The listing builds one solid part. Answer for the finished solid, in the listing's coordinates (mm). Give positions to 0.01 mm unless a question says otherwise; leave off trailing zeros. Write each loop counter-clockwise with the first axis right and the second up, starting at its lowest first coordinate (ties: lowest second). Pieces come first, ordered by that corner, then holes. Notation, with made-up numbers: (-32, 43.25) -> (26, 43.25) arc R22 ccw to (26, 80.25) -> close; hole circle Ø5 at (-15.5, 13). An arc over 180 degrees is marked (long way). One line per question, with ' | ' between items.
Autodesk Inventor part; units mm, degrees
ref_plane "YZ Plane" through (0, 0, 0) normal (1, 0, 0) x (0, 1, 0)
ref_plane "XZ Plane" through (0, 0, 0) normal (0, 1, 0) x (-1, 0, 0)
ref_plane "XY Plane" through (0, 0, 0) normal (0, 0, 1) x (1, 0, 0)
sketch "Szkic1" plane through (0, 0, 0) normal (0, 0, 1) x (1, 0, 0)
  line L0 (-25.3316, -15.5729) -> (26.0684, -15.5729)
  line L1 (26.0684, -15.5729) -> (26.0684, 35.4271)
  line L2 (26.0684, 35.4271) -> (26.0684, 35.4271)
  line L3 (26.0684, 35.4271) -> (26.0684, 55.4271)
  line L4 (26.0684, 55.4271) -> (-5.3316, 55.4271)
  line L5 (-5.3316, 55.4271) -> (-5.3316, 86.8271)
  line L6 (-5.3316, 86.8271) -> (-25.3316, 86.8271)
  line L7 (-25.3316, -15.5729) -> (-25.3316, 86.8271)
  line L8 (-15.6316, 16.9271) -> (16.3684, 16.9271)
  line L9 (16.3684, 16.9271) -> (16.3684, -15.0729)
  line L10 (16.3684, -15.0729) -> (-15.6316, -15.0729)
  line L11 (-15.6316, -15.0729) -> (-15.6316, 16.9271)
  circle A0 centre (0.3684, 0.9271) radius 11
  circle A1 centre (0.3684, 0.9271) radius 16
  point P0 (0, 0)
  point P1 (-10.9453, 12.2408)
  point P2 (11.6821, 12.2408)
  point P3 (11.6821, -10.3866)
  point P4 (-10.9453, -10.3866)
  point P5 (16.0684, 45.4271)
  point P6 (-15.3316, 76.8271)
  point P7 (-15.3316, 45.4271)
  dimension "d0" = 20
  dimension "d1" = 20
  dimension "d2" = 51.4
  dimension "d3" = 51.4
  dimension "d4" = 34.5
  dimension "d5" = 25.7
  dimension "d6" = 51.4
  dimension "d7" = 51
  dimension "d8" = 32
  dimension "d9" = 32
  dimension "d10" = 16
  dimension "d11" = 16
  dimension "d12" = 22
  dimension "d13" = 32
  dimension "d23" = 10
  dimension "d24" = 10
  dimension "d25" = 10
  dimension "d26" = 10
  dimension "d27" = 10
  dimension "d28" = 10
extrude "Wyciągnięcie proste1" add sketch "Szkic1" along normal blind 4 contours L7 L6 L5 L4 L3 L1 L0 | L8 A1 L11 | L8 L9 A1 | A1 | A1 L10 L11 | L9 L10 A1
hole "Otwór1" at (0.3684, 0.9271, 0) at (-10.9453, 12.2408, 0) at (11.6821, 12.2408, 0) at (11.6821, -10.3866, 0) at (-10.9453, -10.3866, 0) direction (0, 0, 1) diameter 4 end through all
hole "Otwór2" at (16.0684, 45.4271, 0) at (-15.3316, 76.8271, 0) at (-15.3316, 45.4271, 0) direction (0, 0, 1) diameter 4 end through all
chamfer "Faza1" distance 51 distance2 9.7 1 edges at (-25.3316, -15.5729, 2) measured on face at (-25.3316, 18.5605, 1.3333)
chamfer "Faza2" distance 51 distance2 9.7 1 edges at (26.0684, -15.5729, 2) measured on face at (26.0684, 31.7605, 1.3333)
fillet "Zaokrąglenie1" radius 2 2 edges at (-15.6316, -15.5729, 2) (16.3684, -15.5729, 2)
fillet "Zaokrąglenie2" radius 6 4 edges at (-5.3316, 55.4271, 2) (26.0684, 55.4271, 2) (-5.3316, 86.8271, 2) (-25.3316, 86.8271, 2)
fillet "Zaokrąglenie3" radius 10 2 edges at (-25.3316, 35.4271, 2) (26.0684, 35.4271, 2)
equation "\"d1\" = d0"
equation "\"d2\" = d6"
equation "\"d3\" = d6"
equation "\"d6\" = 2 * d5"
properties part number "LC_ALU_4mm_Heatbed_Frame_Linear_Bearing_Mounting_Bracket"
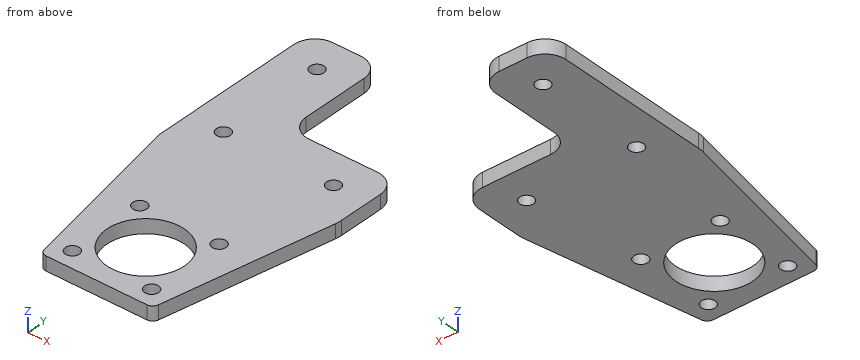
Item 1: Find section C-C (x = 6). Write down the section's boundary in (y, z), then the cut area to 3 significant figures.
Answers below:
outline: (-15.57, 0) -> (-8.52, 0) -> (-8.52, 4) -> (-15.57, 4) -> close; (10.38, 0) -> (55.43, 0) -> (55.43, 4) -> (10.38, 4) -> close | area: 208 mm²
Item 2: Consider line 1 (Y direction, x = -11, z = 0.2); line 2 (Y direction, x = 10, z = 1.55); line 3 (Y direction, x = -14.5, z = 0.7). Determine where each line is inside the solid, lowest interval first. Write a range as [from, to].
Answers below:
line 1: [-15.57, -12.39], [-8.39, 10.24], [14.24, 86.82] | line 2: [-15.57, -11.47], [-9.3, -4.39], [6.24, 11.16], [13.32, 55.43] | line 3: [-15.5, 43.61], [47.25, 75.01], [78.65, 86.83]
Item 3: Find section A-A (z = 1.65). Count the separate pieces of the cut face and the enclosed holes in it, then the cut area to 3 significant figures.
Answers below:
separate pieces: 1 | enclosed holes: 8 | area: 3,300 mm²
Item 4: Find section B-B (y = -6). Write down the section's boundary in (x, z), then the cut area to 3 significant figures.
Answers below:
outline: (-17.45, 0) -> (-8.18, 0) -> (-8.18, 4) -> (-17.45, 4) -> close; (8.91, 0) -> (18.19, 0) -> (18.19, 4) -> (8.91, 4) -> close | area: 74.2 mm²
Item 5: Flat-ended cylindrical pins translate along their axes: pin 1 (1 mm diameter, centred on y = 18, z = 1.5, fed in from +X); pin 2 (1.2 mm diameter, centred on y = 68, z = 1, fed in from +X). Find the tip coordinate at first contact, or state that the pin passes through.
Answers below:
pin 1: x = 22.85 | pin 2: x = -5.33
Item 6: Find section D-D (y = 66.5). Write down the section's boundary in (x, z), then the cut area to 3 significant figures.
Answers below:
outline: (-25.33, 0) -> (-5.33, 0) -> (-5.33, 4) -> (-25.33, 4) -> close | area: 80.0 mm²
